from build123d import *

# Parameters (mm, degrees)
SKETCH1_R           = 18.5
BOSS_EXTRUDE2_DEPTH = 15
SKETCH1_3_R         = 18.5
SKETCH1_3_W         = 25.4
SKETCH1_3_H         = 70
BOSS_EXTRUDE3_DEPTH = 10


with BuildPart() as part:
    # Sketch1 → Boss-Extrude2 (new body)
    with BuildSketch(Plane(origin=(0, 0, 0), x_dir=(1, 0, 0), z_dir=(0, 1, 0))):
        with BuildLine():
            Line((30, 35), (-5.482522909, 28.069591065))
            ThreePointArc((-5.482522909, 28.069591065), (-28.6, 0), (-5.482522909, -28.069591065))
            Line((-5.482522909, -28.069591065), (30, -35))
            Line((30, -35), (30, 35))
        make_face()
        Circle(SKETCH1_R, mode=Mode.SUBTRACT)
    extrude(amount=BOSS_EXTRUDE2_DEPTH)

    # Sketch1_3 → Boss-Extrude3 (add)
    with BuildSketch(Plane(origin=(0, 0, 0), x_dir=(1, 0, 0), z_dir=(0, 1, 0))):
        with BuildLine():
            Line((30, 35), (-5.482522909, 28.069591065))
            ThreePointArc((-5.482522909, 28.069591065), (-28.6, 0), (-5.482522909, -28.069591065))
            Line((-5.482522909, -28.069591065), (30, -35))
            Line((30, -35), (30, 35))
        make_face()
        Circle(SKETCH1_3_R, mode=Mode.SUBTRACT)
        with Locations((42.7, 0)):
            Rectangle(SKETCH1_3_W, SKETCH1_3_H)
    extrude(amount=-BOSS_EXTRUDE3_DEPTH)


solid = part.part
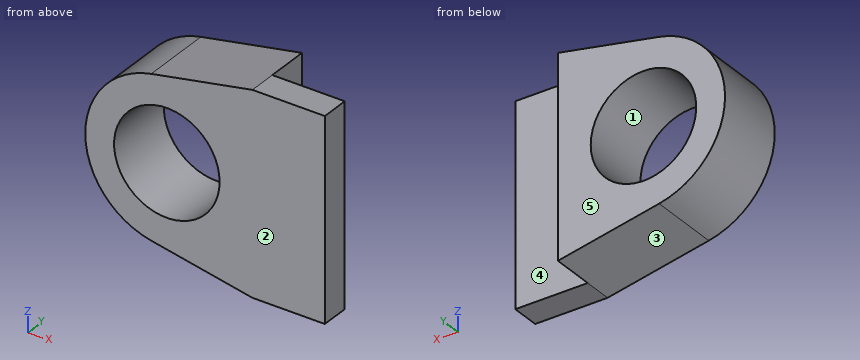
Could you check a few things on this model? Use its own coordinates, in mm. Face numbers are marked on the shaded views. A direction names the side the tool comes from. Round coordinates to 2 decimals unless told otherwise and drop trailing zeros. Write each loop counter-clockwise with the first axis right and the second up, starting at its lowest first coordinate (ties: lowest second). Pieces come first, ordered by that corner, then holes. Notation, with made-up numbers: (31.5, 85) - (80.5, 85) arc R23 ccw to (80.5, 94) - close; hole circle Ø2 at (62.25, -32.75). An arc over 180 degrees is marked (long way). Put each result on its own line as item: value. Start each with the question number.
(1) I need wall thicknesses on probe 1 along Y at (x, z) = (42, 7); probe 2 along Z at (x, y) = (0, -3.25); probe 3 along X at (y, z) = (2.75, 5.5). Which ranges of each line are inside material? Lowest first, please.
(2) I want a section at B-B, the plane y = 1.5. Please give me the cut outline in (x, z), plus the area to 3 significant figures.
(3) I want a section at D-D, the plane x = 16.5. Please give me the cut outline in (y, z).
(4) Thinking about a two-plate mould opening in X: for the marked faces 1, 2 and 3, which applies, released by +X, released by -X, zero draft, split by the parting line, or undercut?
(5) I want a section at A-A, the plane z = 0. Please give me the cut outline in (x, y).
(6) Will these pins go through, and if not, where does the flat tip stop? pin 1 (4 mm diameter, centred on x = 14, y = -4.5, fed in from -Z); pin 2 (6 mm diameter, centred on y = 1.5, z = -9.5, fed in from +X); pin 3 (12 mm diameter, centred on y = 8.5, z = -27.5, fed in from -X); pin 4 (4 mm diameter, centred on x = 46.5, z = -24, fed in from +Y).
(7) I want a section at C-C, the plane x = 0. Please give me the cut outline in (y, z).
(8) For the marked faces 4 and 5, which set-ups out of +Z, -Z, +X, -X, +Y, -Y let a thin tool reach every point of the face, with its end or its side?
Here are the results:
1. probe 1: y = -10 to 0
1. probe 2: z = -29.14 to -18.5, 18.5 to 29.14
1. probe 3: x = -28.07 to -17.66, 17.66 to 30
2. outline: (-5.48, -28.07) - (30, -35) - (30, 35) - (-5.48, 28.07) arc R28.6 ccw to start; hole circle Ø37 at (0, 0)
2. area: 2,140 mm^2
3. outline: (-10, -32.36) - (15, -32.36) - (15, -8.37) - (-10, -8.37) - close; (-10, 8.37) - (15, 8.37) - (15, 32.36) - (-10, 32.36) - close
4. face 1: undercut
4. face 2: zero draft
4. face 3: released by -X
5. outline: (-28.6, -10) - (-18.5, -10) - (-18.5, 15) - (-28.6, 15) - close; (18.5, -10) - (55.4, -10) - (55.4, 0) - (30, 0) - (30, 15) - (18.5, 15) - close
6. pin 1: stops at z = -32.27
6. pin 2: stops at x = 55.4
6. pin 3: stops at x = -18.86
6. pin 4: stops at y = 0
7. outline: (-10, -29.14) - (15, -29.14) - (15, -18.5) - (-10, -18.5) - close; (-10, 18.5) - (15, 18.5) - (15, 29.14) - (-10, 29.14) - close
8. face 4: +Z, -Z, +X, +Y
8. face 5: +Z, -Z, +X, -X, +Y
